from build123d import *

# Parameters (mm, degrees)
EXTRUDE_1_DEPTH     = 5
FILLET_1_R          = 2
SKETCH_2_R          = 2.1
CUT_EXTRUDE_1_DEPTH = 26.019992006


with BuildPart() as part:
    # Эскиз1 → Бобышка-Вытянуть1 (new, symmetric)
    with BuildSketch(Plane(origin=(0, 0, 0), x_dir=(0, 0, -1), z_dir=(1, 0, 0))):
        Polygon((0, 0), (0, 24), (4, 24), (4, 4), (9, 4), (9, 0), (4, 0), (4, -10), (0, -10), align=None)
    extrude(amount=EXTRUDE_1_DEPTH, both=True)

    # Скругление1
    fillet_1_edges = [part.edges().sort_by_distance(p)[0] for p in [
        (-5, 0, -6.5),
        (-5, 4, -6.5),
        (5, 4, -6.5),
        (5, 0, -6.5),
        (5, 24, -2),
        (-5, 24, -2),
        (-5, -10, -2),
        (5, -10, -2),
    ]]
    fillet(fillet_1_edges, radius=FILLET_1_R - 0.0001)  # a hair under: the kernel refuses the full size

    # Эскиз2 → Вырез-Вытянуть1 (cut, through all)
    with BuildSketch(Plane(origin=(0, 0, -4), x_dir=(-1, 0, 0), z_dir=(0, 0, -1))):
        with Locations(Location((0, 14, 0), (0, 0, 90))):
            Circle(SKETCH_2_R)
    extrude(amount=-CUT_EXTRUDE_1_DEPTH, mode=Mode.SUBTRACT)


solid = part.part
Geometry check sheet. Reference: the model listing, model coordinates, mm. A direction names the side the tool comes from. Round coordinates to 2 decimals unless told otherwise and drop trailing zeros. Write each loop counter-clockwise with the first axis right and the second up, starting at its lowest first coordinate (ties: lowest second). Pieces come first, ordered by that corner, then holes. Notation, with made-up numbers: (74.25, 47.5) -> (91.25, 47.5) arc R31 cw to (91.25, 84.5) -> close; hole circle Ø11 at (-27.5, 37.25). An arc over 180 degrees is marked (long way). One line per item, written item: value. Start each with the question number.
(1) Cross-section at C-C, the plane z = -0.75. Record the cut outline in (x, y), and give its area (3 significant figures).
(2) Go/stop test with flat-tipped pins: pin 1 Ø1.5 at (x, y) = (-1.5, -0.5) entering from +Z; pin 2 Ø2 at (x, y) = (-3, 16) entering from -Z; pin 3 Ø1.5 at (x, z) = (1.5, -7) entering from +Y. Record where each tip stops, or that it passes through.
(3) Scan lines: line 1 (X direction, y = 14, z = -2.05); line 2 (Z direction, x = 2, y = -6); line 3 (Y direction, x = -2.5, z = -7.25). Record each from-to range of solid material in increasing order. Write a range as [from, to].
(4) Cross-section at B-B, the plane x = 0. Record the cut outline in (y, z).
(5) Access from +Z, -Z, +X, -X, +Y, -Y to the whole of each face (thin tool, end or side, straight path). Record for faces 1 (the flat face through (0, 4, -6)), 2 (the cylindrical face through (4.4, 3.43, -6.54)), 3 (the flat face through (0, 0, -7)), 4 (the cylindrical face through (-4.4, 3.43, -6.54)), 5 (the cylindrical face through (-4.4, 0.57, -6.46)).
(6) Draft check along X on faces 6 (the flat face through (0, 7, 0)), 7 (the cylindrical face through (4.4, 23.43, -2.03)), 8 (the cylindrical face through (0.09, 11.9, -2.03)). Enter one of: +X half, -X half, draft (parallel to the pull), parting line (faces both ways), or undercut.
(7) Cross-section at A-A, the plane y = 14. Record the cut outline in (x, z), and give its area (3 significant figures).
Answer:
1. outline: (-5, -8) arc R2 ccw to (-3, -10) -> (3, -10) arc R2 ccw to (5, -8) -> (5, 22) arc R2 ccw to (3, 24) -> (-3, 24) arc R2 ccw to (-5, 22) -> close; hole circle Ø4.2 at (0, 14)
1. area: 323 mm²
2. pin 1: z = 0
2. pin 2: z = -4
2. pin 3: y = 4
3. line 1: [-5, -2.1], [2.1, 5]
3. line 2: [-4, 0]
3. line 3: [0, 4]
4. outline: (-10, -4) -> (0, -4) -> (0, -9) -> (4, -9) -> (4, -4) -> (11.9, -4) -> (11.9, 0) -> (-10, 0) -> close; (16.1, -4) -> (24, -4) -> (24, 0) -> (16.1, 0) -> close
5. face 1: -Z, +X, -X, +Y
5. face 2: -Z, +X, +Y
5. face 3: -Z, +X, -X, -Y
5. face 4: -Z, -X, +Y
5. face 5: -Z, -X, -Y
6. face 6: draft
6. face 7: +X half
6. face 8: undercut
7. outline: (-5, -4) -> (-2.1, -4) -> (-2.1, 0) -> (-5, 0) -> close; (2.1, -4) -> (5, -4) -> (5, 0) -> (2.1, 0) -> close
7. area: 23.2 mm²
